Check sheet for the drawn part. Datum: minimum x, y, z corner. Units: mm. A direction names the side the tool comes from. Round coordinates to 2 decimals unless told otherwise and drop trailing zeros. Loops run counter-clockwise (first coordinate to the right, second up) from the corner with the lowest first, then second, coordinate; pieces in that order, holes last.
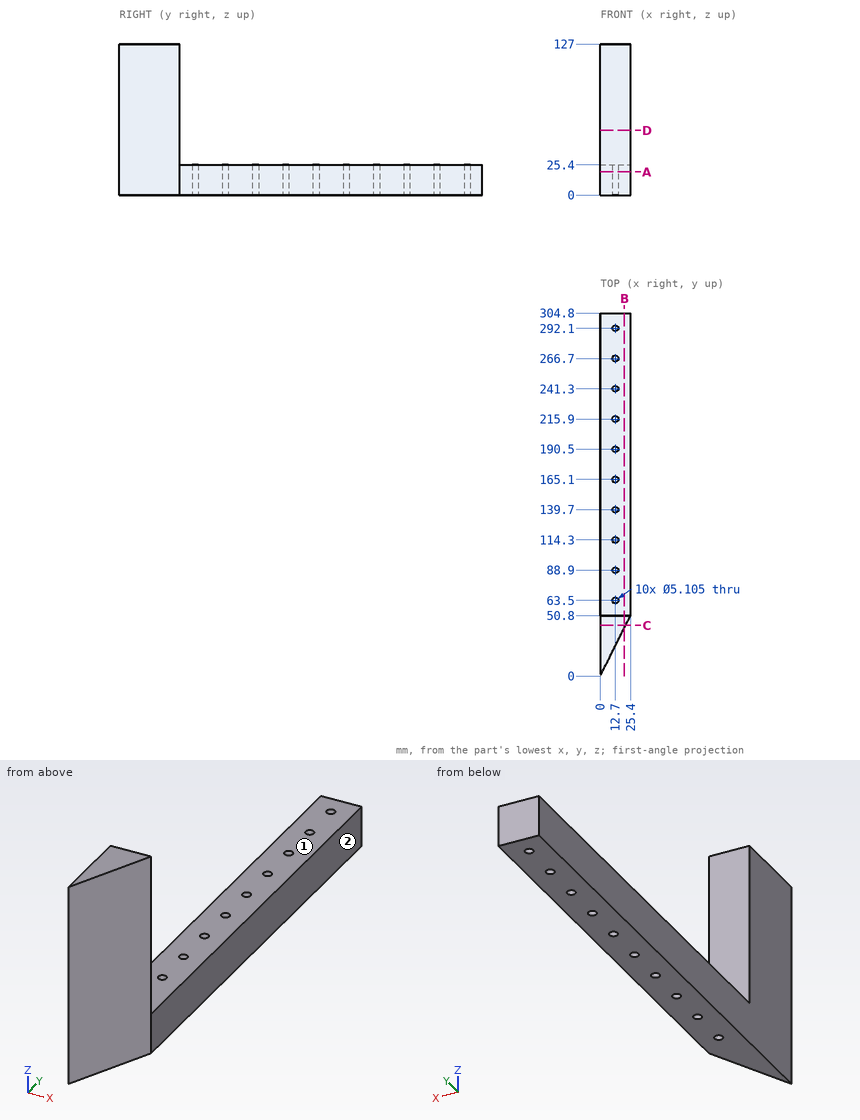
1) Sectioned sample at C-C, the plane y = 42.5. Record the cut outline in (x, z), then the cut area to 3 significant figures.
Report:
outline: (0, 0) - (21.25, 0) - (21.25, 127) - (0, 127) - close
area: 2,700 mm2
2) Sectioned sample at D-D, the plane z = 54.5. Record the cut outline in (x, y), then the cut area to 3 significant figures.
Report:
outline: (0, 0) - (25.4, 50.8) - (0, 50.8) - close
area: 645 mm2
3) Access from +Z, -Z, +X, -X, +Y, -Y to the whole of each face (thin tool, end or side, straight path). Record for the marked faces 1 and 2.
Report:
face 1: +Z, +X, -X, +Y
face 2: +Z, -Z, +X, +Y, -Y
4) Gauge pin test, flat ends, axial feed: pin 1 (8 mm diameter, centred on x = 12, z = 28.5, fed in from -Y); pin 2 (10 mm diameter, centred on x = 10.5, z = 59, fed in from +Y); pin 3 (6.5 mm diameter, centred on x = 12.7, y = 190.5, fed in from +Z). Record the tip position at first contact, or that the pin passes through.
Report:
pin 1: stops at y = 16
pin 2: stops at y = 50.8
pin 3: stops at z = 25.4
5) Sectioned sample at A-A, the plane z = 19.5. State how many separate pieces and enclosed holes the cut face has, then the cut area to 3 significant figures.
Report:
separate pieces: 1
enclosed holes: 10
area: 6,890 mm2
6) Sectioned sample at B-B, the plane x = 20.25. Record the cut outline in (y, z).
Report:
outline: (40.5, 0) - (304.8, 0) - (304.8, 25.4) - (50.8, 25.4) - (50.8, 127) - (40.5, 127) - close
7) Scan lines: line 1 along X through (y, z) = (241, 12) (1 decimal); line 2 along Z through (x, y) = (24.25, 175); line 3 along Y through (x, z) = (17, 38). Record each from-to range of solid material in increasing order.
Report:
line 1: x = 0 to 10.2, 15.2 to 25.4
line 2: z = 0 to 25.4
line 3: y = 34 to 50.8
